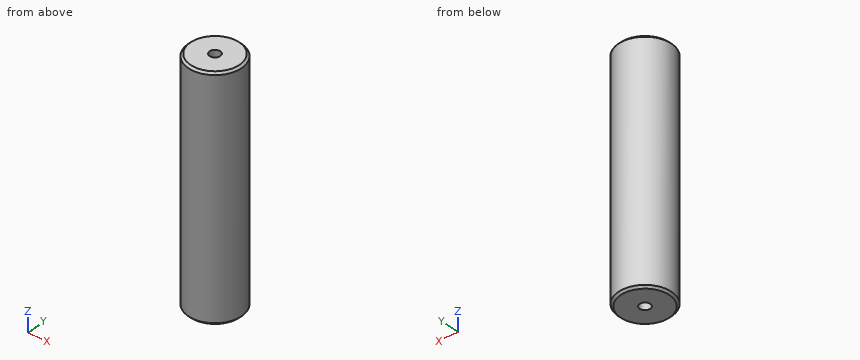
from build123d import *

# Parameters (mm, degrees)
SKETCH1_R           = 12.5
BOSS_EXTRUDE1_DEPTH = 55
CHAMFER1_SIZE       = 1


with BuildPart() as part:
    # Sketch1 → Boss-Extrude1 (new body, symmetric)
    with BuildSketch(Plane.XY):
        Circle(SKETCH1_R)
    extrude(amount=BOSS_EXTRUDE1_DEPTH, both=True)

    # Chamfer1
    chamfer1_edges = [part.edges().sort_by_distance(p)[0] for p in [
        (-12.5, 0, -55),
        (-12.5, 0, 55),
    ]]
    chamfer(chamfer1_edges, length=CHAMFER1_SIZE)

    # Sketch4 → M6 Tapped Hole1 (revolve, cut)
    with BuildSketch(Plane(origin=(0, 0, 55), x_dir=(0, -1, 0), z_dir=(1, 0, 0))):
        Polygon((0, 0), (0, 16.502151548), (2.5, 15), (2.5, 0), align=None)
    m6_tapped_hole1 = revolve(axis=Axis((0, 0, 61.35), (0, 0, -1)), mode=Mode.SUBTRACT)

    # Mirror1: M6 Tapped Hole1 across plane
    add(m6_tapped_hole1.mirror(Plane.XY), mode=Mode.SUBTRACT)


solid = part.part
Part model, mm, in its own coordinate system. Give positions to 0.01 mm unless a question says otherwise; leave off trailing zeros. Loops run counter-clockwise (first coordinate to the right, second up) from the corner with the lowest first, then second, coordinate; pieces in that order, holes last. Notation, with made-up numbers: M -9.75,13.5 L 30.25,13.5 A12 ccw 30.25,36.5 Z; hole C -26,27 d11. An arc over 180 degrees is marked long. Put each result on its own line as item: value. Start each with the question number.
1) Probe probe 1 along Y at (x, z) = (0, 46.5); probe 2 along Y at (x, z) = (-7.25, -27.5); probe 3 along Y at (x, z) = (2.25, -19.5). List the from-to ranges inside material, lowest first.
2) Flat gauge pins, fed straight in: pin 1 (3 mm diameter, centred on y = -1.5, z = 27.5, fed in from -X); pin 2 (3 mm diameter, centred on y = -3.5, z = 4.5, fed in from +X); pin 3 (12 mm diameter, centred on x = -6.5, z = 26, fed in from -Y); pin 4 (1.5 mm diameter, centred on y = -1.5, z = 26, fed in from +X). Where does each tip first touch, or does it go through?
3) Saw through at B-B (z = 4.5). List the corners of the cut face in (x, y).
4) Saw through at A-A (z = -46). List the corners of the cut face in (x, y), then the cut area to 3 significant figures.
Numbers:
1. probe 1: -12.5 to -2.5, 2.5 to 12.5
1. probe 2: -10.18 to 10.18
1. probe 3: -12.3 to 12.3
2. pin 1: x = -12.5
2. pin 2: x = 12.34
2. pin 3: y = -12.49
2. pin 4: x = 12.48
3. outline: C 0,0 d25
4. outline: C 0,0 d25; hole C 0,0 d5
4. area: 471 mm^2
